Source: CAD feature listing. Evaluate the final solid. Frame: model axes, mm. A direction names the side the tool comes from. Coordinates: 2 decimals unless noted, no trailing zeros. Write each loop counter-clockwise with the first axis right and the second up, starting at its lowest first coordinate (ties: lowest second). Pieces come first, ordered by that corner, then holes. Notation, with made-up numbers: (77, 60.5) - (126, 60.5) arc R21 ccw to (126, 79.5) - close; hole circle Ø10 at (58, -15). An arc over 180 degrees is marked (long way). One line per question, with ' | ' between items. Start each with the question number.
Q1. Access query for faces 4 (the face through (3.2, 0.1, 53)), 5 (the face through (2.44, 0.54, -45.34)). Directions: +Z, -Z, +X, -X, +Y, -Y. A direction counts if a zero-diameter tool reaches every point of the face in a straight line with its end or side. Return the directions, or none.
Q2. Cut plane A-A, the plane z = 30. Return loops of the section in (x, y).
Q3. Draft query along Y for faces 1 (the face through (-7.493, 0.33, 0.742)), 2 (the face through (2.44, 0.54, 45.34)), 3 (the face through (3.2, 0.1, -53)). Return one class per face: +Y half, -Y half, draft (parallel to the pull), parting line (faces both ways), or undercut.
Q4. Cut plane C-C, the plane x = 4.5. Return loops of the section in (y, z), plus the area to 3 significant figures.
Q5. Cut plane B-B, the plane y = 5. Return loops of the section in (x, z), plus the area to 3 significant figures.
Q6. Line query: line 1 (Y direction, x = 0, z = 43.25); line 2 (X direction, y = -4.75, z = -22.5); line 3 (X direction, y = 4.25, z = 45). Output: solid intervals per line, ascending.
Q7. Contact query for flat-ended pins moving along their axis: P1, Ø3, axis at x = -2, z = 16, coming from the +Y side; P2, Ø1.5, axis at y = -1.5, z = -5.5, coming from the -X side; P3, Ø3, axis at y = 2.5, z = -2.5, coming from the -X side. Output: stop coordinate, or through.
```python
from build123d import *

# Parameters (mm, degrees)
SKETCH1_R           = 7.5
BOSS_EXTRUDE1_DEPTH = 53


with BuildPart() as part:
    # Sketch1 → Boss-Extrude1 (new body, symmetric)
    with BuildSketch(Plane.XY):
        Circle(SKETCH1_R)
    extrude(amount=BOSS_EXTRUDE1_DEPTH, both=True)

    # Sketch3 → M6x1.0 Tapped Hole1 (revolve, cut)
    with BuildSketch(Plane(origin=(0, 0, 53), x_dir=(0, -1, 0), z_dir=(1, 0, 0))):
        Polygon((0, 0), (0, 16.502151548), (2.5, 15), (2.5, 0.525), (3.025, 0), align=None)
    m6x1_0_tapped_hole1 = revolve(axis=Axis((0, 0, 59.35), (0, 0, -1)), mode=Mode.SUBTRACT)

    # Mirror1: M6x1.0 Tapped Hole1 across plane
    add(m6x1_0_tapped_hole1.mirror(Plane.XY), mode=Mode.SUBTRACT)


solid = part.part
```
Reply:
1) face 4: +Z, +X, -X, +Y, -Y | face 5: -Z
2) outline: circle Ø15 at (0, 0)
3) face 1: parting line | face 2: undercut | face 3: draft
4) outline: (-6, -53) - (6, -53) - (6, 53) - (-6, 53) - close | area: 1,270 mm^2
5) outline: (-5.59, -53) - (5.59, -53) - (5.59, 53) - (-5.59, 53) - close | area: 1,190 mm^2
6) line 1: y = -7.5 to -2.5, 2.5 to 7.5 | line 2: x = -5.8 to 5.8 | line 3: x = -6.18 to 6.18
7) P1: stops at y = 7.48 | P2: stops at x = -7.46 | P3: stops at x = -7.43
